CAD build for the part. Positions are in the model's coordinates, mm. A direction names the side the tool comes from. Give positions to 0.01 mm unless a question says otherwise; leave off trailing zeros. Write each loop counter-clockwise with the first axis right and the second up, starting at its lowest first coordinate (ties: lowest second). Pieces come first, ordered by that corner, then holes. Notation, with made-up numbers: (25.5, 58) - (73.5, 58) arc R9 cw to (73.5, 64) - close; hole circle Ø3 at (44, -0.5). An arc over 180 degrees is marked (long way). Answer as a JSON object with one key per item and string values.
from build123d import *

# Parameters (mm, degrees)
BOSS_EXTRU_1_DEPTH = 52
ESQUISSE2_W        = 22
ESQUISSE2_H        = 82
BOSS_EXTRU_2_DEPTH = 1
ESQUISSE3_W        = 18
ESQUISSE3_H        = 82
BOSS_EXTRU_3_DEPTH = 1
BOSS_EXTRU_4_START = -1
BOSS_EXTRU_4_DEPTH = 76
ESQUISSE6_W        = 39
ESQUISSE6_H        = 82
BOSS_EXTRU_5_DEPTH = 1


with BuildPart() as part:
    # Esquisse1 → Boss.-Extru.1 (new body)
    with BuildSketch(Plane.XY):
        Polygon((22, 82), (22, 81), (21, 81), (1, 81), (1, 1), (21, 1), (22, 1), (22, 0), (0, 0), (0, 82), align=None)
    extrude(amount=BOSS_EXTRU_1_DEPTH)

    # Esquisse2 → Boss.-Extru.2 (add)
    with BuildSketch(Plane.XY.offset(52)):
        with Locations((11, 41)):
            Rectangle(ESQUISSE2_W, ESQUISSE2_H)
    extrude(amount=BOSS_EXTRU_2_DEPTH)

    # Esquisse3 → Boss.-Extru.3 (add)
    with BuildSketch(Plane(origin=(22, 0, 0), x_dir=(0, 0, -1), z_dir=(1, 0, 0))):
        with Locations((-44, 41)):
            Rectangle(ESQUISSE3_W, ESQUISSE3_H)
    extrude(amount=BOSS_EXTRU_3_DEPTH)

    # Esquisse5 → Boss.-Extru.4 (add)
    with BuildSketch(Plane(origin=(23, 0, 0), x_dir=(0, 0, -1), z_dir=(1, 0, 0)).offset(BOSS_EXTRU_4_START)):
        Polygon((-39, 0), (0, 0), (0, 1), (-35, 1), (-35, 81), (0, 81), (0, 82), (-39, 82), align=None)
    extrude(amount=BOSS_EXTRU_4_DEPTH)

    # Esquisse6 → Boss.-Extru.5 (add)
    with BuildSketch(Plane(origin=(98, 0, 0), x_dir=(0, 0, -1), z_dir=(1, 0, 0))):
        with Locations((-19.5, 41)):
            Rectangle(ESQUISSE6_W, ESQUISSE6_H)
    extrude(amount=BOSS_EXTRU_5_DEPTH)


solid = part.part
(1) Probe L1, parallel to Y at x = 21, z = 6.5; L2, parallel to X at y = 54.5, z = 37; L3, parallel to X at y = 77, z = 42. List the from-to ranges inside material, lowest first. Write a range as [from, to].
Answer key:
{"L1": "y = [0, 1], [81, 82]", "L2": "x = [0, 1], [22, 99]", "L3": "x = [0, 1], [22, 23]"}
(2) Saw through at B-B, the plane x = 41. Give the cut face in (y, z).
Answer key:
{"outline": "(0, 0) - (1, 0) - (1, 35) - (81, 35) - (81, 0) - (82, 0) - (82, 39) - (0, 39) - close"}
(3) Flat gauge pins, fed straight in: P1, Ø6, axis at x = 32, y = 18.5, coming from the -Z side; P2, Ø15.5, axis at y = 55, z = 49.5, coming from the +X side; P3, Ø17, axis at x = 11.5, y = 27, coming from the -Z side. Where does each tip first touch, or does it go through?
Answer key:
{"P1": "stops at z = 35", "P2": "stops at x = 23", "P3": "stops at z = 52"}
(4) 3-axis set-ups, long thin cutter, end or side, ignore diameter. For faces 4 (the face through (1, 42, 26)), 5 (the face through (49, 82, 21)), 6 (the face through (23, 42, 46)): which of +Z, -Z, +X, -X, +Y, -Y reach the whole face in a straight line?
Answer key:
{"face 4": "-Z", "face 5": "+Z, -Z, +X, -X, +Y", "face 6": "+Z, +X, +Y, -Y"}
(5) Saw through at D-D, the plane x = 16. Give the cut face in (y, z), and give its area (3 significant figures).
Answer key:
{"outline": "(0, 0) - (1, 0) - (1, 52) - (81, 52) - (81, 0) - (82, 0) - (82, 53) - (0, 53) - close", "area": "186 mm²"}
(6) Pull direction X, two halves, no side cores. Call faces 1 (the face through (60, 40, 39)), 2 (the face through (11, 42, 52)), 3 (the face through (99, 42, 20)): pulls with the +X half, pulls with the -X half, needs draft (parallel to the pull), parting line crosses it, or undercut.
Answer key:
{"face 1": "needs draft", "face 2": "undercut", "face 3": "pulls with the +X half"}
(7) Saw through at C-C, the plane y = 36. Give the cut face in (x, z), and give its area (3 significant figures).
Answer key:
{"outline": "(0, 0) - (1, 0) - (1, 52) - (22, 52) - (22, 35) - (98, 35) - (98, 0) - (99, 0) - (99, 39) - (23, 39) - (23, 53) - (0, 53) - close", "area": "431 mm²"}
(8) Saw through at A-A, the plane z = 12. Give the cut face in (x, y).
Answer key:
{"outline": "(0, 0) - (99, 0) - (99, 82) - (0, 82) - close; hole (1, 1) - (98, 1) - (98, 81) - (1, 81) - close"}
